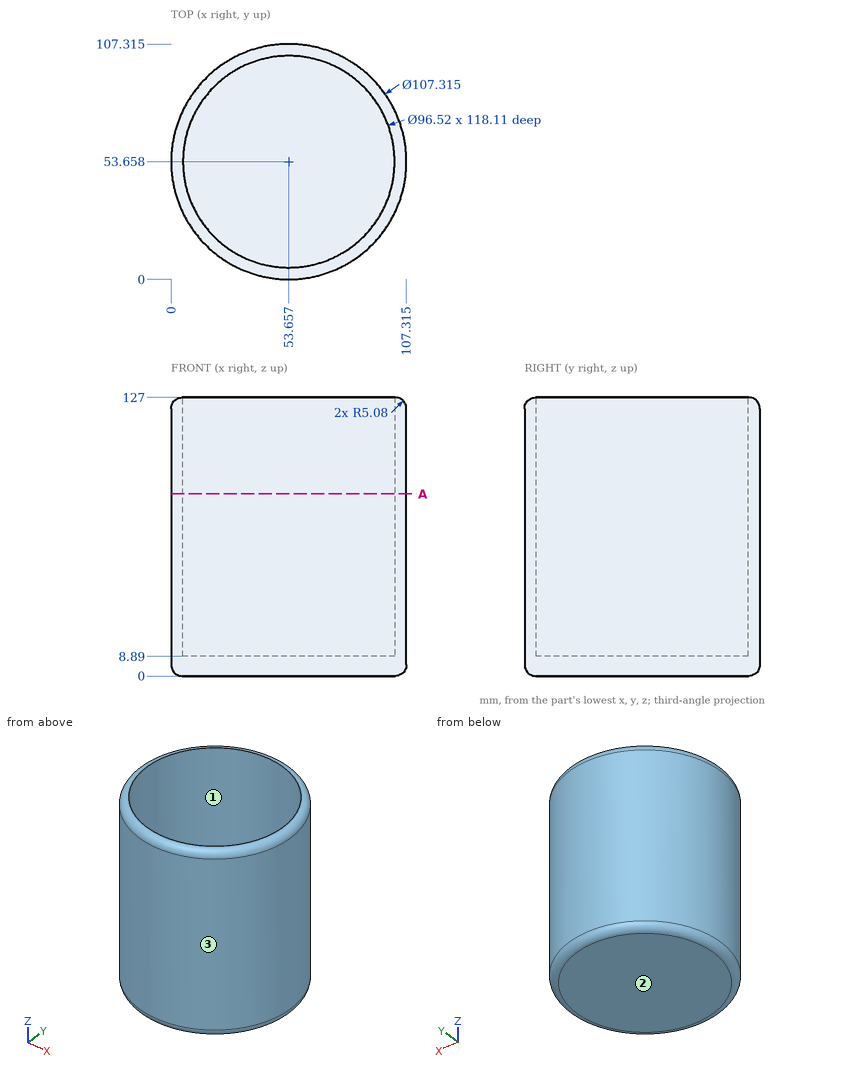
Answer from the drawing. Dimensions are ordinates in mm from the lowest x, y and z of the part. Give positions to 0.01 mm unless a question says otherwise; leave off trailing zeros. Write each loop counter-clockwise with the first axis right and the second up, starting at its lowest first coordinate (ties: lowest second). Pieces come first, ordered by that corner, then holes.
1) Section A-A (z = 83) is taken. Write down the section's boundary in (x, y) (1 decimal), and give its area (3 significant figures).
2) Given P1, Ø1.5, axis at x = 84.5, z = 36, coming from the +Y side; P2, Ø2, axis at y = 68.5, z = 26, coming from the -X side; P3, Ø1, axis at x = 94.5, z = 44, coming from the +Y side (1 decimal), each flat-ended and moving along its own axis, determine where each tip first touches the part or whether it passes through.
3) Find the intervals of material crossed by L1, parallel to X at y = 52, z = 35 (1 decimal); L2, parallel to Z at x = 44, y = 60; L3, parallel to Y at x = 84, z = 33 (1 decimal), in increasing order.
4) For a pull along Y with two mould halves and no side action, classify the marked faces 1, 2 and 3 as pulls with the +Y half, pulls with the -Y half, needs draft (parallel to the pull), parting line crosses it, or undercut.
Response:
1. outline: circle Ø107.3 at (53.7, 53.7); hole circle Ø96.5 at (53.7, 53.7)
1. area: 1,730 mm2
2. P1: stops at y = 98.08
2. P2: stops at x = 1.82
2. P3: stops at y = 89
3. L1: x = 0 to 5.4, 101.9 to 107.3
3. L2: z = 0 to 8.89
3. L3: y = 9.4 to 16.1, 91.2 to 97.9
4. face 1: undercut
4. face 2: needs draft
4. face 3: parting line crosses it
